Geometry: see drawing. Coordinates: mm, zero at the bounding-box minimum. Round coordinates to 2 decimals unless told otherwise and drop trailing zeros. Write each loop counter-clockwise with the first axis right and the second up, starting at its lowest first coordinate (ties: lowest second). Pieces come first, ordered by that corner, then holes.
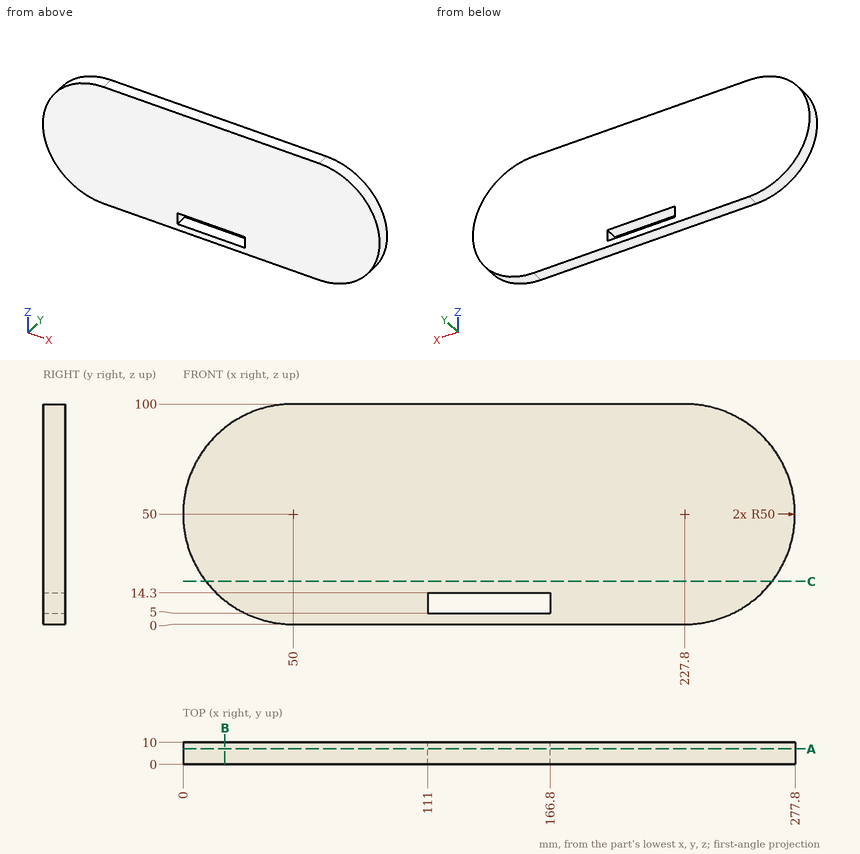
1) Material intervals for line 1 (Z direction, x = 114, y = 2); line 2 (X direction, y = 5, z = 48); line 3 (X direction, y = 1, z = 79), sorted ascending.
Taken from the geometry:
line 1: z = 0 to 5, 14.3 to 100
line 2: x = 0.04 to 277.76
line 3: x = 9.27 to 268.53
2) Section query C-C on z = 19.5. Return the cut outline in (x, y).
Taken from the geometry:
outline: (10.38, 0) - (267.42, 0) - (267.42, 10) - (10.38, 10) - close
3) Section query A-A on y = 7. Return the cut outline in (x, z).
Taken from the geometry:
outline: (50, 0) - (227.8, 0) arc R50 ccw to (227.8, 100) - (50, 100) arc R50 ccw to start; hole (111, 5) - (166.8, 5) - (166.8, 14.3) - (111, 14.3) - close
4) Section query B-B on x = 19. Return the cut outline in (y, z), then the cut area to 3 significant figures.
Taken from the geometry:
outline: (0, 10.77) - (10, 10.77) - (10, 89.23) - (0, 89.23) - close
area: 785 mm2
5) Contact query for flat-ended pins moving along their axis: P1, Ø6, axis at x = 177.5, z = 48, coming from the -Y side; P2, Ø4, axis at y = 5.5, z = 44, coming from the -X side; P3, Ø5, axis at y = 2, z = 87.5, coming from the -X side; P4, Ø1.5, axis at y = 8, z = 21.5, coming from the +X side. Output: stop coordinate, or through.
Taken from the geometry:
P1: stops at y = 0
P2: stops at x = 0.16
P3: stops at x = 14.29
P4: stops at x = 269.39
